Design review of the part built by this model. Coordinates are the model's own, in mm. Face numbers are marked on the shaded views. A direction names the side the tool comes from. Give positions to 0.01 mm unless a question says otherwise; leave off trailing zeros. Order: outer loops, then holes, each group sorted by start corner. A loop starts at its lowest first (then second) coordinate and runs counter-clockwise, first axis right, second up.
```python
from build123d import *

# Parameters (mm, degrees)
CUT_EXTRUDE1_DEPTH = 0.25


with BuildPart() as part:
    # Sketch2 → Revolve1 (revolve)
    with BuildSketch(Plane(origin=(0, 0, 0), x_dir=(0, 0, -1), z_dir=(1, 0, 0)), mode=Mode.PRIVATE) as revolve1_sk:
        Polygon((0, 0), (0, 2.8), (1.65, 1.5), (6, 1.5), (6, 0), align=None)
    revolve(revolve1_sk.sketch.rotate(Axis((0, 0, 0), (0, 0, -1)), 90), axis=Axis((0, 0, 0), (0, 0, -1)))

    # Sketch3 → Cut-Extrude1 (cut)
    with BuildSketch(Plane.XY):
        Polygon((-0.25, 2.8), (-0.25, 0.25), (-2.8, 0.25), (-3.256058343, -0.027319636), (-2.8, -0.25), (-0.25, -0.25), (-0.25, -2.8), (0.125, -3.416695886), (0.25, -2.8), (0.25, -0.25), (2.8, -0.25), (3.211130591, 0), (2.8, 0.25), (0.25, 0.25), (0.25, 2.8), (0, 3.10316335), align=None)
    extrude(amount=-CUT_EXTRUDE1_DEPTH, mode=Mode.SUBTRACT)


solid = part.part
```
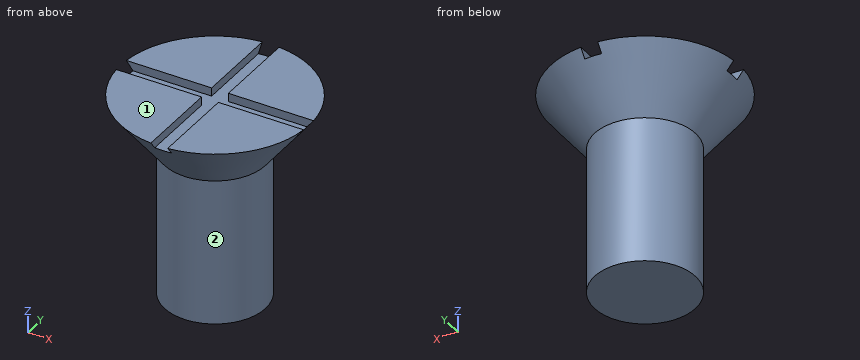
1. Machinability: for the marked faces 1 and 2, which of the approach directions +Z, -Z, +X, -X, +Y, -Y give a long, thin tool a straight path to every point of the face, cutting with its end or side? Answer none if there is none.
Recorded:
face 1: +Z, +X, -X, +Y, -Y
face 2: -Z
2. Take a section at A-A (y = 0). State the section outline as (x, z) points, then the cut area to 3 significant figures.
Recorded:
outline: (-2.6, -0.25) - (-1.5, -1.65) - (-1.5, -6) - (1.5, -6) - (1.5, -1.65) - (2.6, -0.25) - close
area: 18.8 mm2
3. Take a section at C-C (z = -0.5). State the section outline as (x, y) points.
Recorded:
outline: circle Ø4.81 at (0, 0)
4. For line 1 along Z through (x, y) = (0.2, 0.7); line 2 along Z through (x, y) = (-1.9, -0.35); line 3 along Y through (x, z) = (1.15, -2.25), list the stretches that pass through material, from the lowest coordinate up.
Recorded:
line 1: z = -6 to -0.25
line 2: z = -1.1 to 0
line 3: y = -0.96 to 0.96
